from build123d import *

# Parameters (mm, degrees)
SKETCH_1_W          = 142
SKETCH_1_H          = 142
EXTRUDE_1_DEPTH     = 113
SKETCH_2_R          = 7
CUT_EXTRUDE_1_DEPTH = 113
SKETCH_3_R          = 18
CUT_EXTRUDE_2_DEPTH = 103
SKETCH_4_OUTSIDE_W  = 190.086
SKETCH_4_OUTSIDE_H  = 190.086
SKETCH_4_OUTSIDE_R  = 95
CUT_EXTRUDE_3_DEPTH = 231.427862899
EXTRUDE_2_DEPTH     = 113
SKETCH_6_R          = 7.5
CUT_EXTRUDE_4_DEPTH = 113


with BuildPart() as part:
    # 草图1 → 拉伸1 (new body)
    with BuildSketch(Plane.XY):
        with Locations((71, -71)):
            Rectangle(SKETCH_1_W, SKETCH_1_H)
    extrude(amount=EXTRUDE_1_DEPTH)

    # 草图2 → 切除-拉伸1 (cut)
    with BuildSketch(Plane.XY.offset(113)):
        with Locations((14, -14)):
            Circle(SKETCH_2_R)
        with Locations((128, -14)):
            Circle(SKETCH_2_R)
        with Locations((14, -128)):
            Circle(SKETCH_2_R)
        with Locations((128, -128)):
            Circle(SKETCH_2_R)
    extrude(amount=-CUT_EXTRUDE_1_DEPTH, mode=Mode.SUBTRACT)

    # 草图3 → 切除-拉伸2 (cut)
    with BuildSketch(Plane.XY.offset(113)):
        with Locations((71, -71)):
            Circle(SKETCH_3_R)
    extrude(amount=-CUT_EXTRUDE_2_DEPTH, mode=Mode.SUBTRACT)

    # 草图4 outside → 切除-拉伸3 (cut, through all)
    with BuildSketch(Plane(origin=(0, 0, 0), x_dir=(-1, 0, 0), z_dir=(0, 0, -1))):
        with Locations((-71, -71)):
            Rectangle(SKETCH_4_OUTSIDE_W, SKETCH_4_OUTSIDE_H)
        with Locations((-71, -71)):
            Circle(SKETCH_4_OUTSIDE_R, mode=Mode.SUBTRACT)
    extrude(amount=-CUT_EXTRUDE_3_DEPTH, mode=Mode.SUBTRACT)

    # 草图5 → 拉伸2 (add)
    with BuildSketch(Plane(origin=(0, 0, 0), x_dir=(-1, 0, 0), z_dir=(0, 0, -1))):
        Polygon((11, -55), (0, -52.5), (0, -55), (0, -87), (0, -89.5), (11, -87), align=None)
    extrude(amount=-EXTRUDE_2_DEPTH)

    # 草图6 → 切除-拉伸4 (cut)
    with BuildSketch(Plane.ZY.offset(11)):
        with Locations(Location((24.5, -71, 0), (0, 0, 270))):
            Circle(SKETCH_6_R)
        with Locations(Location((88.5, -71, 0), (0, 0, 270))):
            Circle(SKETCH_6_R)
    extrude(amount=-CUT_EXTRUDE_4_DEPTH, mode=Mode.SUBTRACT)


solid = part.part
Geometry: final body of the model. Coordinates: model frame, mm. A direction names the side the tool comes from. Round coordinates to 2 decimals unless told otherwise and drop trailing zeros. Order: outer loops, then holes, each group sorted by start corner. A loop starts at its lowest first (then second) coordinate and runs counter-clockwise, first axis right, second up. Notation, with made-up numbers: (43.5, 74.5) -> (80.5, 74.5) arc R30 cw to (80.5, 111.5) -> close; hole circle Ø8 at (58.5, 7.5). An arc over 180 degrees is marked (long way). Put each result on its own line as item: value. Start each with the question number.
Q1. Pull-direction query (X, two-part tool) for faces 1 (the cylindrical face through (67.098, -88.572, 62.221)), 2 (the cylindrical face through (138.23, -138.12, 55.71)), 3 (the flat face through (71, -71, 10)), 4 (the flat face through (102, -71, 89)); classes: +X half, -X half, draft (parallel to the pull), parting line (faces both ways), or undercut.
Q2. Line query: probe 1 along Z at (x, y) = (21, -71); probe 2 along Y at (x, z) = (28, 88.5); probe 3 along Y at (x, z) = (13.5, 13). Output: solid intervals per line, ascending.
Q3. First-contact query: pin 1 (11 mm diameter, centred on x = 66.5, y = -78, fed in from +Z); pin 2 (13.5 mm diameter, centred on y = -71, z = 88.5, fed in from -X); pin 3 (1 mm diameter, centred on x = 38, y = -55, fed in from -Z); pin 4 (12.5 mm diameter, centred on x = 128, y = -128, fed in from +Z). Flat tips, straight axial feed; report the tip coordinate or a pass-through.
Q4. Reachability of faces 5 (the flat face through (0, -112, 56)), 6 (the cylindrical face through (94.579, -74.461, 17.846)), 7 (the cylindrical face through (121, -14, 57)) from +Z, -Z, +X, -X, +Y, -Y: full face, straight path, thin tool, end or side. Return the list, or none.
Q5. Section A-A on y = -14. Return the cut outline in (x, z).
Q6. Section B-B on z = 60.5. Return the cut outline in (x, y).
Q7. Section D-D on x = 59.5. Return the cut outline in (y, z), and give its area (3 significant figures).
Q8. Section C-C on z = 24.5. Return the cut outline in (x, y), and give its area (3 significant figures).
Ans:
1. face 1: undercut
1. face 2: +X half
1. face 3: undercut
1. face 4: -X half
2. probe 1: z = 0 to 17, 32 to 81, 96 to 113
2. probe 2: y = -142 to -78.5, -63.5 to 0
2. probe 3: y = -142 to -134.98, -121.02 to -20.98, -7.02 to 0
3. pin 1: stops at z = 10
3. pin 2: stops at x = 102
3. pin 3: stops at z = 0
3. pin 4: passes through
4. face 5: +Z, -Z, -X, -Y
4. face 6: -X
4. face 7: +Z, -Z
5. outline: (0, 0) -> (7, 0) -> (7, 113) -> (0, 113) -> close; (21, 0) -> (121, 0) -> (121, 113) -> (21, 113) -> close; (135, 0) -> (142, 0) -> (142, 113) -> (135, 113) -> close
6. outline: (-11, -87) -> (0, -89.5) -> (0, -134.12) arc R95 ccw to (7.88, -142) -> (134.12, -142) arc R95 ccw to (142, -134.12) -> (142, -7.88) arc R95 ccw to (134.12, 0) -> (7.88, 0) arc R95 ccw to (0, -7.88) -> (0, -52.5) -> (-11, -55) -> close; hole circle Ø14 at (14, -128); hole circle Ø14 at (14, -14); hole circle Ø36 at (71, -71); hole circle Ø14 at (128, -128); hole circle Ø14 at (128, -14)
7. outline: (-142, 0) -> (0, 0) -> (0, 113) -> (-57.15, 113) -> (-57.15, 10) -> (-84.85, 10) -> (-84.85, 113) -> (-142, 113) -> close
7. area: 13,200 mm2
8. outline: (-11, -87) -> (0, -89.5) -> (0, -134.12) arc R95 ccw to (7.88, -142) -> (134.12, -142) arc R95 ccw to (142, -134.12) -> (142, -7.88) arc R95 ccw to (134.12, 0) -> (7.88, 0) arc R95 ccw to (0, -7.88) -> (0, -52.5) -> (-11, -55) -> (-11, -63.5) -> (54.64, -63.5) arc R18 cw to (87.36, -63.5) -> (102, -63.5) -> (102, -78.5) -> (87.36, -78.5) arc R18 cw to (54.64, -78.5) -> (-11, -78.5) -> close; hole circle Ø14 at (14, -128); hole circle Ø14 at (14, -14); hole circle Ø14 at (128, -128); hole circle Ø14 at (128, -14)
8. area: 17,600 mm2
